from build123d import *

# Parameters (mm, degrees)
SKETCH1_R               = 30
EXTRUDE1_DEPTH          = 3.4
SKETCH2_R               = 33.4
SKETCH2_R_2             = 30
EXTRUDE2_DEPTH          = 8.3
EXTRUDE3_START          = 9.8
SKETCH3_R               = 33.4
SKETCH3_R_2             = 30
EXTRUDE3_DEPTH          = 9.8
EXTRUDE4_START          = -18.1
SKETCH4_R               = 34.5
SKETCH4_R_2             = 33.4
EXTRUDE4_DEPTH          = 18.1
SKETCH6_R               = 34.5
SKETCH6_R_2             = 33
EXTRUDE5_DEPTH          = 1
EXTRUDE6_START          = -1
SKETCH8_R               = 34.5
SKETCH8_R_2             = 33
EXTRUDE6_DEPTH          = 1
SKETCH9_R               = 3.175
EXTRUDE7_DEPTH          = 5.08
EXTRUDE8_START          = 17.78
SKETCH10_R              = 3.175
SKETCH10_R_2            = 1.905
EXTRUDE8_DEPTH          = 17.78
SKETCH13_R              = 2.6
EXTRUDE11_DEPTH         = 10
CIRPATTERN1_COUNT       = 7
CUT_EXTRUDE1_REACH      = 55.189
CUT_EXTRUDE1_END_RADIUS = 3.175
SKETCH14_R              = 0.635
CUT_EXTRUDE2_REACH      = 57.408
SKETCH15_R              = 1.905


with BuildPart() as part:
    # Sketch1 → Extrude1 (new body)
    with BuildSketch(Plane.XY):
        Circle(SKETCH1_R)
    extrude(amount=EXTRUDE1_DEPTH)



with BuildPart() as body_2:
    # Sketch2 → Extrude2 (new body)
    with BuildSketch(Plane.XY.offset(3.4)):
        with Locations(Location((0, 0, 0), (0, 0, 180))):
            Circle(SKETCH2_R)
        Circle(SKETCH2_R_2, mode=Mode.SUBTRACT)
    extrude(amount=EXTRUDE2_DEPTH)


with BuildPart() as part_1:
    add(part.part)

    add(body_2.part)  # Extrude3 merges body 2
    # Sketch3 → Extrude3 (add)
    with BuildSketch(Plane(origin=(0, 0, 3.4), x_dir=(-1, 0, 0), z_dir=(0, 0, -1)).offset(EXTRUDE3_START)):
        with Locations(Location((0, 0, 0), (0, 0, 180))):
            Circle(SKETCH3_R)
        with Locations(Location((0, 0, 0), (0, 0, 180))):
            Circle(SKETCH3_R_2, mode=Mode.SUBTRACT)
    extrude(amount=-EXTRUDE3_DEPTH)

    # Sketch4 → Extrude4 (add)
    with BuildSketch(Plane.XY.offset(11.7).offset(EXTRUDE4_START)):
        Circle(SKETCH4_R)
        Circle(SKETCH4_R_2, mode=Mode.SUBTRACT)
    extrude(amount=EXTRUDE4_DEPTH)

    # Sketch6 → Extrude5 (cut)
    with BuildSketch(Plane(origin=(0, 0, -6.4), x_dir=(-1, 0, 0), z_dir=(0, 0, -1))):
        with Locations(Location((0, 0, 0), (0, 0, 180))):
            Circle(SKETCH6_R)
        Circle(SKETCH6_R_2, mode=Mode.SUBTRACT)
    extrude(amount=-EXTRUDE5_DEPTH, mode=Mode.SUBTRACT)

    # Sketch8 → Extrude6 (cut)
    with BuildSketch(Plane.XY.offset(11.7).offset(EXTRUDE6_START)):
        Circle(SKETCH8_R)
        with Locations(Location((0, 0, 0), (0, 0, 180))):
            Circle(SKETCH8_R_2, mode=Mode.SUBTRACT)
    extrude(amount=EXTRUDE6_DEPTH, mode=Mode.SUBTRACT)

    # Sketch9 → Extrude7 (add)
    with BuildSketch(Plane(origin=(0, 0, 0), x_dir=(-1, 0, 0), z_dir=(0, 0, -1))):
        with Locations(Location((0, 0, 0), (0, 0, 180))):
            Circle(SKETCH9_R)
    extrude(amount=EXTRUDE7_DEPTH)

    # Sketch10 → Extrude8 (add)
    with BuildSketch(Plane.XY.offset(3.4).offset(EXTRUDE8_START)):
        Circle(SKETCH10_R)
        with Locations(Location((0, 0, 0), (0, 0, 180))):
            Circle(SKETCH10_R_2, mode=Mode.SUBTRACT)
    extrude(amount=-EXTRUDE8_DEPTH)

    # Sketch13 → Extrude11 (cut, symmetric)
    with BuildSketch(Plane.XY.offset(3.4)):
        with Locations((-19, 0)):
            Circle(SKETCH13_R)
    extrude11 = extrude(amount=EXTRUDE11_DEPTH, both=True, mode=Mode.SUBTRACT)

    # CirPattern1: Extrude11 ×7 about axis
    cirpattern1_axis = Axis((0, 0, 0), (0, 0, 1))
    for i in range(1, CIRPATTERN1_COUNT):
        add(extrude11.rotate(cirpattern1_axis, i * 360 / CIRPATTERN1_COUNT), mode=Mode.SUBTRACT)

    # Cut-Extrude1: up to this cylinder (the profile starts inside it)
    cut_extrude1_end = Plane(origin=(0, 0, 16.1), z_dir=(0, 0, -1)) * Cylinder(CUT_EXTRUDE1_END_RADIUS, 117.728, mode=Mode.PRIVATE)
    # Sketch14 → Cut-Extrude1 (cut, up to the surface)
    with BuildSketch(Plane(origin=(0, 0, 0), x_dir=(0, 0, -1), z_dir=(1, 0, 0)), mode=Mode.PRIVATE) as cut_extrude1_sk1:
        with Locations(Location((-16.1, 0, 0), (0, 0, 180))):
            Circle(SKETCH14_R)
    cut_extrude1_tool1 = extrude(cut_extrude1_sk1.sketch, amount=CUT_EXTRUDE1_REACH, mode=Mode.PRIVATE) & cut_extrude1_end
    add(cut_extrude1_tool1.solids().sort_by_distance((0, 0, 16.1))[0], mode=Mode.SUBTRACT)

    # Sketch15 → Cut-Extrude2 (cut, up to next)
    with BuildSketch(Plane(origin=(0, 0, -5.08), x_dir=(-1, 0, 0), z_dir=(0, 0, -1)), mode=Mode.PRIVATE) as cut_extrude2_sk1:
        Circle(SKETCH15_R)
    cut_extrude2_tool1 = extrude(cut_extrude2_sk1.sketch, amount=-CUT_EXTRUDE2_REACH, mode=Mode.PRIVATE) & part_1.part
    add(cut_extrude2_tool1.solids().sort_by_distance((0, 0, -5.08))[0], mode=Mode.SUBTRACT)


solid = part_1.part
Geometry: final body of the model. Coordinates: model frame, mm. A direction names the side the tool comes from. Give positions to 0.01 mm unless a question says otherwise; leave off trailing zeros. Loops run counter-clockwise (first coordinate to the right, second up) from the corner with the lowest first, then second, coordinate; pieces in that order, holes last. Notation, with made-up numbers: (-29.75, 44.25) - (-11.75, 44.25) arc R9 cw to (-11.75, 48.25) - close; hole circle Ø1 at (28, 78). An arc over 180 degrees is marked (long way). Answer as CSV lines item,"result". Start each with the question number.
1. Ray query, L1, parallel to Y at x = 0, z = 9.5 (3 decimals); L2, parallel to X at y = 1, z = 9.5; L3, parallel to Z at x = 21.5, y = -9.5. Return the intervals inside material, ascending.
2. Reachability of faces 1 (the face through (-10.213, -16.878, 1.724)), 2 (the face through (-30.5, -12.6, -5.9)), 3 (the face through (6, 0, 3.4)) from +Z, -Z, +X, -X, +Y, -Y: full face, straight path, thin tool, end or side. Return the list, or none.
3. Pin query (flat end, axial travel): P1, Ø3, axis at x = -2, y = 20, coming from the +Z side; P2, Ø4, axis at y = -3, z = 9, coming from the +X side; P3, Ø6, axis at x = 17.12, y = 8.24, coming from the -Z side; P4, Ø1.5, axis at x = 24.5, y = 26.5, coming from the -Z side. Return the tip coordinate at first contact, or that it passes through.
4. Draft query along X for faces 4 (the face through (32.907, 10.363, 2.537)), 5 (the face through (15, -27, -6.4)), 6 (the face through (4.694, -21.081, 1.724)), 7 (the face through (1.5, 2.8, -2.5)). Return one class per face: released by +X, released by -X, zero draft, split by the parting line, or undercut.
5. Section D-D, the plane y = -26.5. Return loops of the section in (x, z), plus the area to 3 significant figures.
6. Section C-C, the plane x = -19. Return loops of the section in (y, z), plus the area to 3 significant figures.
7. Section B-B, the plane y = -15. Return loops of the section in (x, z), plus the area to 3 significant figures.
Answers:
1,L1,"y = -34.5 to -30, -3.175 to -1.905, 1.905 to 3.175, 30 to 34.5"
1,L2,"x = -34.49 to -29.98, -3.01 to -1.62, 1.62 to 3.01, 29.98 to 34.49"
1,L3,"z = 0 to 3.4"
2,face 1,"+Z, -Z"
2,face 2,"-Z"
2,face 3,"+Z"
3,P1,"stops at z = 3.4"
3,P2,"stops at x = 34.49"
3,P3,"stops at z = 0"
3,P4,"passes through"
4,face 4,"split by the parting line"
4,face 5,"zero draft"
4,face 6,"undercut"
4,face 7,"undercut"
5,outline,"(-22.09, -5.4) - (-19.67, -5.4) - (-19.67, -6.4) - (-14.06, -6.4) - (-14.06, 0) - (14.06, 0) - (14.06, -6.4) - (19.67, -6.4) - (19.67, -5.4) - (22.09, -5.4) - (22.09, 10.7) - (19.67, 10.7) - (19.67, 11.7) - (14.06, 11.7) - (14.06, 3.4) - (-14.06, 3.4) - (-14.06, 11.7) - (-19.67, 11.7) - (-19.67, 10.7) - (-22.09, 10.7) - close"
5,area,"377 mm2"
6,outline,"(-28.8, -5.4) - (-26.98, -5.4) - (-26.98, -6.4) - (-23.22, -6.4) - (-23.22, 0) - (-2.6, 0) - (-2.6, 3.4) - (-23.22, 3.4) - (-23.22, 11.7) - (-26.98, 11.7) - (-26.98, 10.7) - (-28.8, 10.7) - close; (2.6, 0) - (23.22, 0) - (23.22, -6.4) - (26.98, -6.4) - (26.98, -5.4) - (28.8, -5.4) - (28.8, 10.7) - (26.98, 10.7) - (26.98, 11.7) - (23.22, 11.7) - (23.22, 3.4) - (2.6, 3.4) - close"
6,area,"335 mm2"
7,outline,"(-31.07, -5.4) - (-29.39, -5.4) - (-29.39, -6.4) - (-25.98, -6.4) - (-25.98, 0) - (-14.44, 0) - (-14.44, 3.4) - (-25.98, 3.4) - (-25.98, 11.7) - (-29.39, 11.7) - (-29.39, 10.7) - (-31.07, 10.7) - close; (-9.25, 0) - (25.98, 0) - (25.98, -6.4) - (29.39, -6.4) - (29.39, -5.4) - (31.07, -5.4) - (31.07, 10.7) - (29.39, 10.7) - (29.39, 11.7) - (25.98, 11.7) - (25.98, 3.4) - (-9.25, 3.4) - close"
7,area,"336 mm2"
